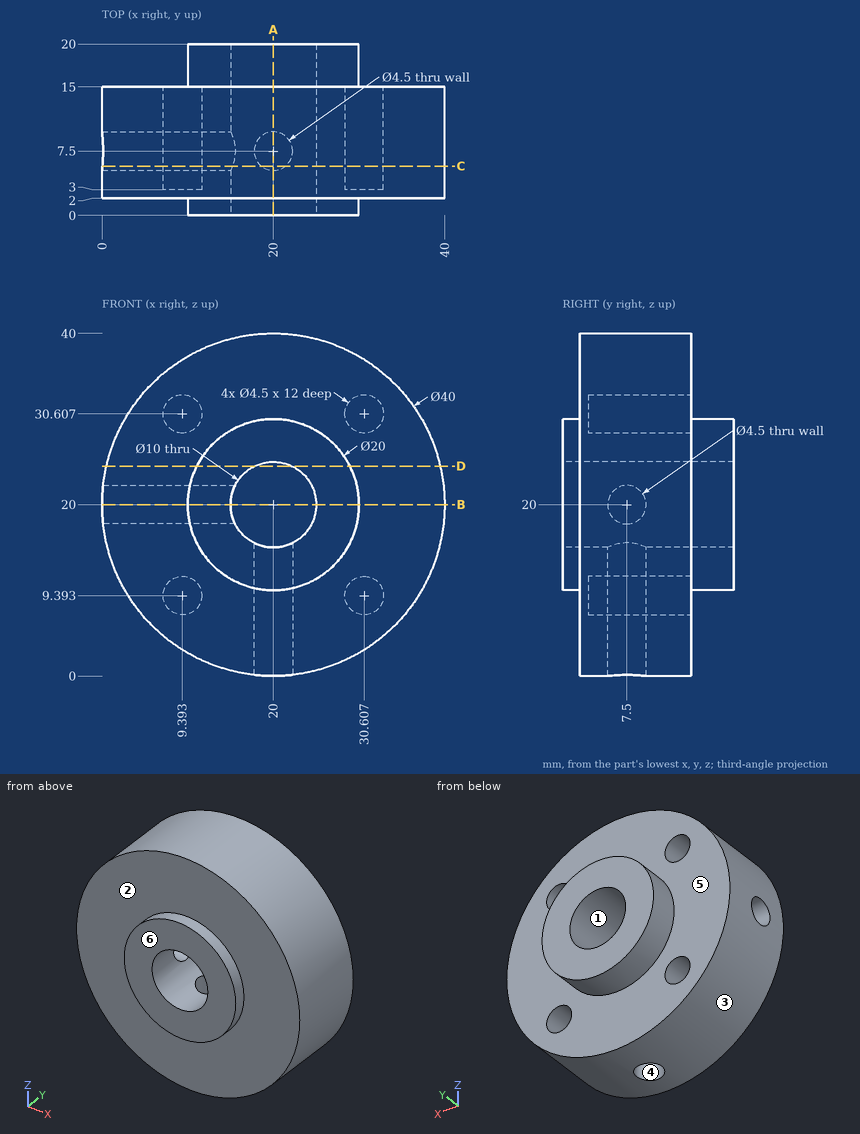
The drawing under review shows one solid part. Ordinate dimensions are in mm from its lowest x, y, z. A direction names the side the tool comes from. Coordinates: 2 decimals unless noted, no trailing zeros. Write each loop counter-clockwise with the first axis right and the second up, starting at its lowest first coordinate (ties: lowest second). Pieces come first, ordered by that corner, then holes. Notation, with made-up numbers: M -15,-25.5 L 40,-25.5 A18 cw 40,-17.5 Z; hole C 67.5,67 d11. An arc over 180 degrees is marked long. Answer as a JSON object with one key per item and string values.
Item 1: Add section B-B, the plane z = 20. Give the boundary of the cut face in (x, y).
Outcome:
{"outline": "M 0,2 L 10,2 L 10,0 L 15,0 L 15,5.25 L 0,5.25 Z; M 0,9.75 L 15,9.75 L 15,20 L 10,20 L 10,15 L 0,15 Z; M 25,0 L 30,0 L 30,2 L 40,2 L 40,15 L 30,15 L 30,20 L 25,20 Z"}
Item 2: Draft analysis for pull direction Z (two halves, no side actions). For the marked faces 1, 2 and 3, state which applies: pulls with the +Z half, pulls with the -Z half, needs draft (parallel to the pull), parting line crosses it, or undercut.
Outcome:
{"face 1": "undercut", "face 2": "needs draft", "face 3": "parting line crosses it"}
Item 3: Wall thickness on probe 1 along Y at (x, z) = (26, 6); probe 2 along Z at (x, y) = (2.5, 8.5) (1 decimal); probe 3 along Z at (x, y) = (32.5, 11.75) (1 decimal): over which ranges is each line inside the solid? List them lowest first.
Outcome:
{"probe 1": "2 to 15", "probe 2": "10.3 to 18, 22 to 29.7", "probe 3": "4.4 to 8.2, 10.6 to 29.4, 31.8 to 35.6"}
Item 4: Insertion check: pin 1 Ø1.3 at (x, z) = (10.5, 31.5) entering from +Y; pin 2 Ø6 at (x, z) = (30.61, 9.39) entering from -Y; pin 3 Ø4 at (x, y) = (16.5, 6) entering from +Z; pin 4 Ø8 at (x, z) = (20, 20) entering from +Y. Each pin has a flat end and moves straight along its axis. Give the tip position at first contact, or say it passes through.
Outcome:
{"pin 1": "y = 3", "pin 2": "y = 2", "pin 3": "z = 39.94", "pin 4": "through"}
Item 5: Machinability: for the marked faces 4, 5 and 6, which of the approach directions +Z, -Z, +X, -X, +Y, -Y give a long, thin tool a straight path to every point of the face, cutting with its end or side? Answer none if there is none.
Outcome:
{"face 4": "-Z", "face 5": "+Y", "face 6": "+Z, -Z, +X, -X, -Y"}
Item 6: Add section D-D, the plane z = 24.5. Give the boundary of the cut face in (x, y).
Outcome:
{"outline": "M 0.51,2 L 11.07,2 L 11.07,0 L 17.82,0 L 17.82,20 L 11.07,20 L 11.07,15 L 0.51,15 Z; M 22.18,0 L 28.93,0 L 28.93,2 L 39.49,2 L 39.49,15 L 28.93,15 L 28.93,20 L 22.18,20 Z"}
Item 7: Add section A-A, the plane x = 20. Give the boundary of the cut face in (y, z).
Outcome:
{"outline": "M 0,10 L 2,10 L 2,0 L 5.25,0 L 5.25,15 L 0,15 Z; M 0,25 L 20,25 L 20,30 L 15,30 L 15,40 L 2,40 L 2,30 L 0,30 Z; M 9.75,0 L 15,0 L 15,10 L 20,10 L 20,15 L 9.75,15 Z"}
Item 8: Add section C-C, the plane y = 5.75. State how many separate pieces and enclosed holes the cut face has, and give its area (3 significant figures).
Outcome:
{"separate pieces": "2", "enclosed holes": "4", "area": "1,030 mm²"}
